Check sheet for the drawn part. Datum: minimum x, y, z corner. Units: mm. Coordinates: 2 decimals unless noted, no trailing zeros. Loops run counter-clockwise (first coordinate to the right, second up) from the corner with the lowest first, then second, coordinate; pieces in that order, holes last. Notation, with made-up numbers: (-22, -27) -> (16, -27) arc R13 ccw to (16, -15) -> close; hole circle Ø9 at (85.5, 28). An arc over 180 degrees is marked (long way). Use CSV: the item, a comma, the result in double quotes. Start each with the question number.
1. Sectioned sample at B-B, the plane x = 266.7. Record the cut outline in (y, z).
2. Thickness scan on L1, parallel to Z at x = 190.5, y = 3.5; L2, parallel to X at y = 3.25, z = 5; L3, parallel to X at y = 3.5, z = 7. Record the ranges inside material, lowest first.
3. Sectioned sample at A-A, the plane z = 6.35. Record the cut outline in (x, y), and give its area (3 significant figures).
4. Sectioned sample at C-C, the plane y = 4. Count the separate pieces of the cut face and the enclosed holes in it, and give its area (3 significant figures).
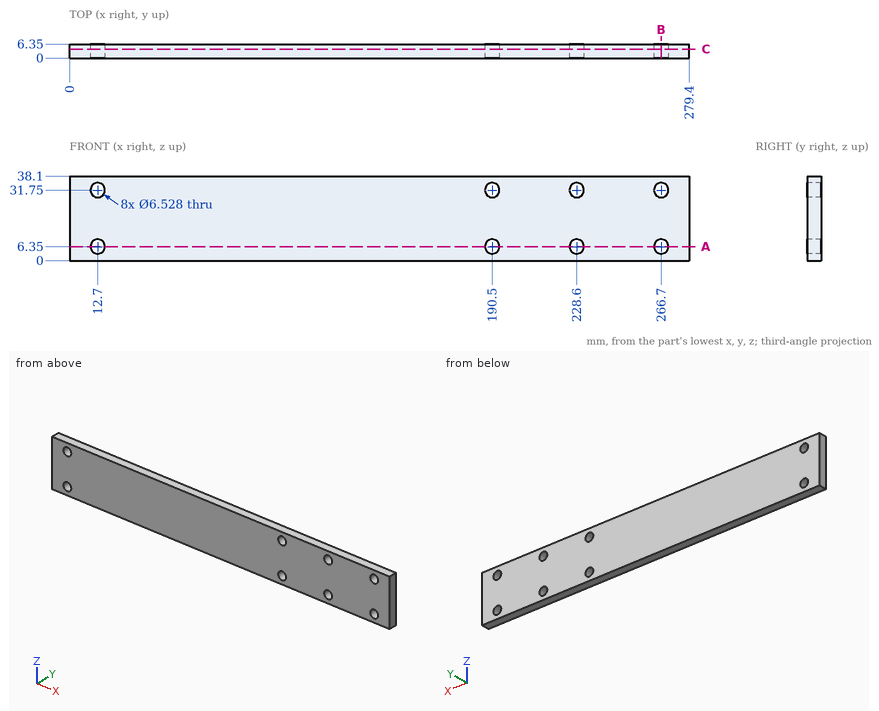
Completed:
1,outline,"(0, 0) -> (6.35, 0) -> (6.35, 3.09) -> (0, 3.09) -> close; (0, 9.61) -> (6.35, 9.61) -> (6.35, 28.49) -> (0, 28.49) -> close; (0, 35.01) -> (6.35, 35.01) -> (6.35, 38.1) -> (0, 38.1) -> close"
2,L1,"0 to 3.09, 9.61 to 28.49, 35.01 to 38.1"
2,L2,"0 to 9.73, 15.67 to 187.53, 193.47 to 225.63, 231.57 to 263.73, 269.67 to 279.4"
2,L3,"0 to 9.5, 15.9 to 187.3, 193.7 to 225.4, 231.8 to 263.5, 269.9 to 279.4"
3,outline,"(0, 0) -> (9.44, 0) -> (9.44, 6.35) -> (0, 6.35) -> close; (15.96, 0) -> (187.24, 0) -> (187.24, 6.35) -> (15.96, 6.35) -> close; (193.76, 0) -> (225.34, 0) -> (225.34, 6.35) -> (193.76, 6.35) -> close; (231.86, 0) -> (263.44, 0) -> (263.44, 6.35) -> (231.86, 6.35) -> close; (269.96, 0) -> (279.4, 0) -> (279.4, 6.35) -> (269.96, 6.35) -> close"
3,area,"1,610 mm²"
4,separate pieces,"1"
4,enclosed holes,"8"
4,area,"10,400 mm²"
